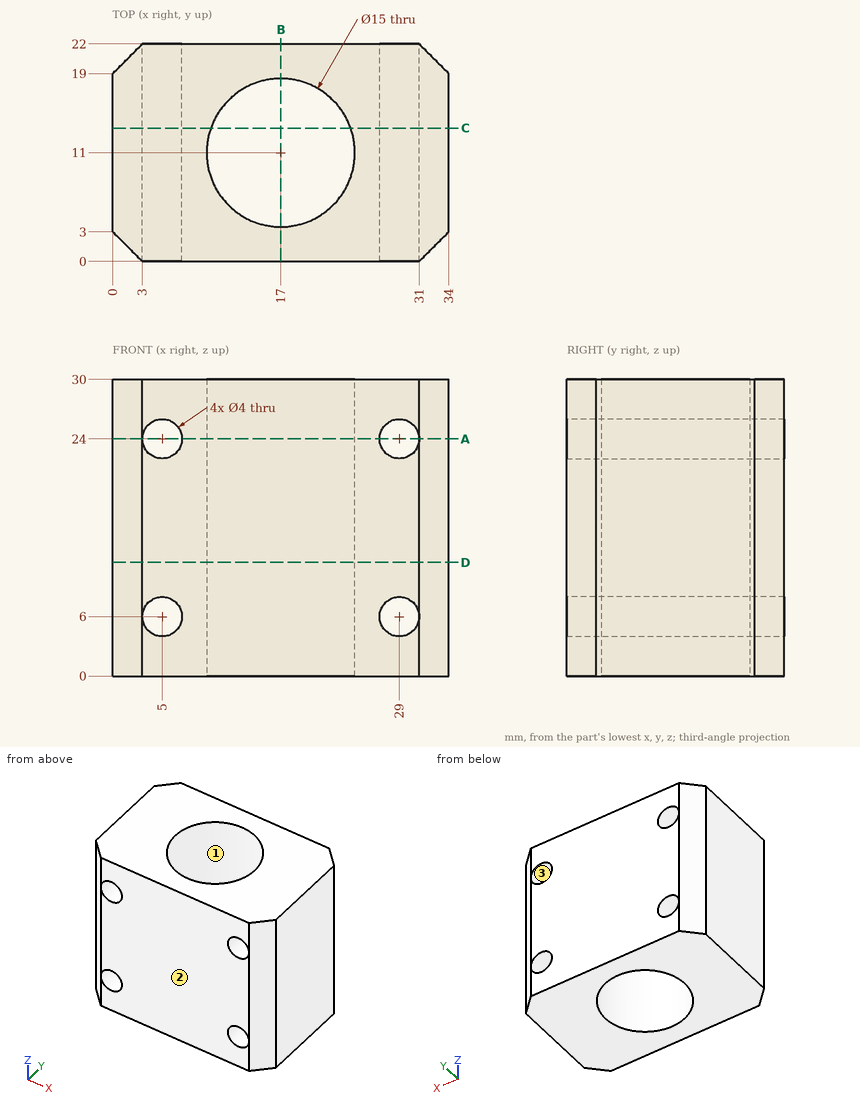
Part print with two shaded views. Sizes in mm from the minimum x, y, z corner. Round coordinates to 2 decimals unless told otherwise and drop trailing zeros. Order: outer loops, then holes, each group sorted by start corner. A loop starts at its lowest first (then second) coordinate and runs counter-clockwise, first axis right, second up. Notation, with made-up numbers: M 15.5,-37 L 28.5,-37 A17 ccw 28.5,-30 Z; hole C -37.75,31.5 d2. An arc over 180 degrees is marked long. Put each result on its own line as item: value. Start each with the question number.
1. Slice it at B-B on x = 17. List the corners of the cut face in (y, z), then the cut area to 3 significant figures.
2. Slice it at A-A on z = 24. State how many separate pieces and enclosed holes the cut face has, then the cut area to 3 significant figures.
3. Slice it at D-D on z = 11.5. List the corners of the cut face in (x, y), then the cut area to 3 significant figures.
4. Two-plate mould, pull along Y, no slides. Class the marked faces 1, 2 and 3: +Y half, -Y half, draft (parallel to the pull), parting line (faces both ways), or undercut.
5. Slice it at C-C on y = 13.5. List the corners of the cut face in (x, z).
6. Drop flat-ended pins along their axis: pin 1 (3.5 mm diameter, centred on x = 29, z = 24, fed in from +Y); pin 2 (5 mm diameter, centred on x = 20, y = 18, fed in from -Z). Give the stop position or say it passes through.
7. Drill centre lines: probe 1 along X at (y, z) = (20.5, 23.5); probe 2 along Z at (x, y) = (27.5, 20.5); probe 3 along Y at (x, z) = (17, 10.75). Where is each one in solid material? Low to high. Write a range as [from, to].
Findings:
1. outline: M 0,0 L 3.5,0 L 3.5,30 L 0,30 Z; M 18.5,0 L 22,0 L 22,30 L 18.5,30 Z
1. area: 210 mm2
2. separate pieces: 3
2. enclosed holes: 1
2. area: 377 mm2
3. outline: M 0,3 L 3,0 L 31,0 L 34,3 L 34,19 L 31,22 L 3,22 L 0,19 Z; hole C 17,11 d15
3. area: 553 mm2
4. face 1: undercut
4. face 2: -Y half
4. face 3: draft
5. outline: M 0,0 L 9.93,0 L 9.93,30 L 0,30 Z; M 24.07,0 L 34,0 L 34,30 L 24.07,30 Z; hole C 5,6 d4; hole C 5,24 d4; hole C 29,6 d4; hole C 29,24 d4
6. pin 1: through
6. pin 2: z = 0
7. probe 1: [1.5, 3.06], [6.94, 27.06], [30.94, 32.5]
7. probe 2: [0, 4.68], [7.32, 22.68], [25.32, 30]
7. probe 3: [0, 3.5], [18.5, 22]
